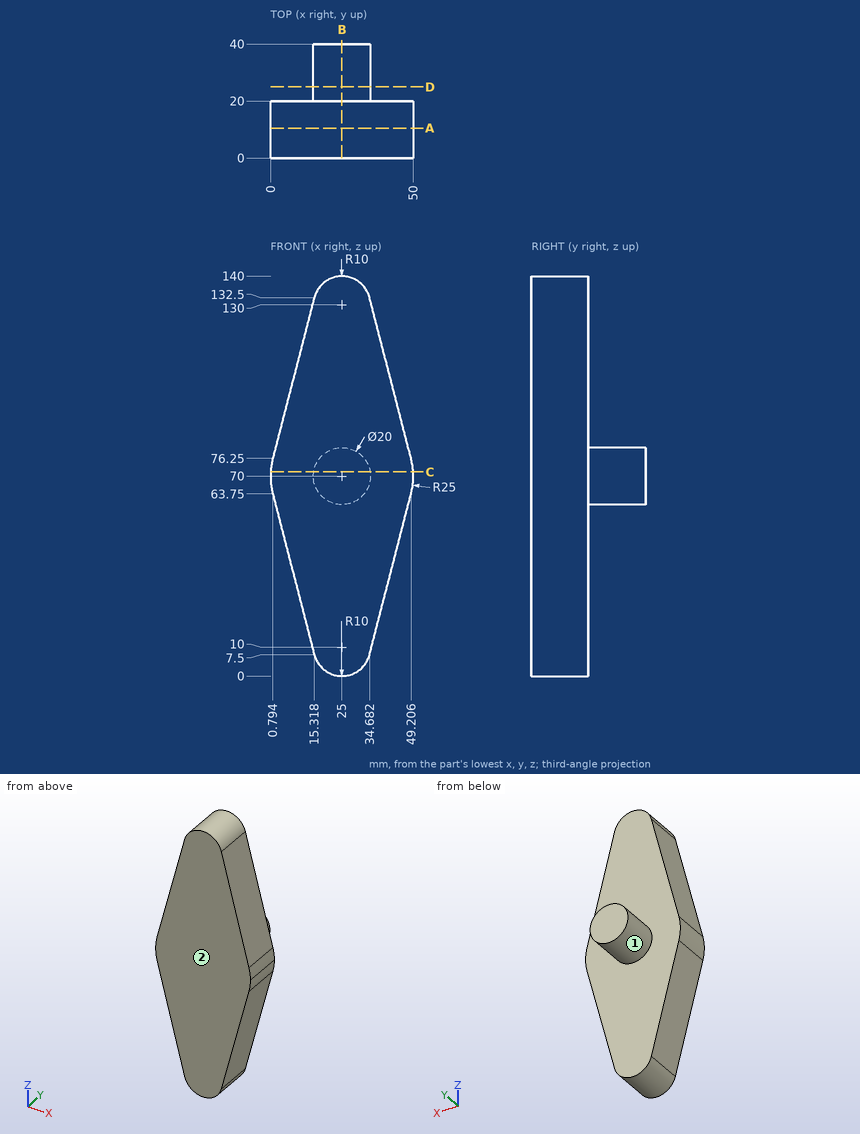
Here's the drawing with two shaded views (mm, measured from the low corner). I have some questions. A direction names the side the tool comes from. Round coordinates to 2 decimals unless told otherwise and drop trailing zeros. Loops run counter-clockwise (first coordinate to the right, second up) from the corner with the lowest first, then second, coordinate; pieces in that order, holes last.
Item 1: Suppose I cut it at A-A, the plane y = 10.5. Write out the boundary of the cut face in (x, z).
Item 2: Will these pins go through, and if not, where does the flat tip stop? pin 1 Ø1.5 at (x, z) = (15, 46.5) entering from -Y; pin 2 Ø6 at (y, z) = (16.5, 108) entering from +X; pin 3 Ø1.5 at (x, y) = (15.5, 30) entering from -Z; pin 4 Ø2 at (y, z) = (15, 23.5) entering from +X.
Item 3: Suppose I cut it at B-B, the plane x = 25. Write out the boundary of the cut face in (y, z), then the cut area to 3 significant figures.
Item 4: Suppose I cut it at C-C, the plane z = 71.5. Write out the boundary of the cut face in (x, y) (1 decimal), then the cut area to 3 significant figures.
Item 5: Which directions (+Z, -Z, +X, -X, +Y, -Y) give clear straight access to the entire face, cutting with the end or side of a thin tool? Please do the marked faces 1 and 2.
Item 6: Please list where these lines run through material, in increasing order: L1, parallel to Y at x = 11.5, z = 94.5; L2, parallel to Z at x = 20, y = 33; L3, parallel to X at y = 3, z = 65 (1 decimal).
Item 7: Suppose I cut it at D-D, the plane y = 25. Write out the boundary of the cut face in (x, z).
Reported:
1. outline: (0.79, 63.75) - (15.32, 7.5) arc R10 ccw to (34.68, 7.5) - (49.21, 63.75) arc R25 ccw to (50, 70) arc R25 ccw to (49.21, 76.25) - (34.68, 132.5) arc R10 ccw to (15.32, 132.5) - (0.79, 76.25) arc R25 ccw to start
2. pin 1: stops at y = 0
2. pin 2: stops at x = 41.78
2. pin 3: stops at z = 65.16
2. pin 4: stops at x = 39.07
3. outline: (0, 0) - (20, 0) - (20, 60) - (40, 60) - (40, 80) - (20, 80) - (20, 140) - (0, 140) - close
3. area: 3,200 mm2
4. outline: (0, 0) - (50, 0) - (50, 20) - (34.9, 20) - (34.9, 40) - (15.1, 40) - (15.1, 20) - (0, 20) - close
4. area: 1,390 mm2
5. face 1: +Y
5. face 2: +Z, -Z, +X, -X, -Y
6. L1: y = 0 to 20
6. L2: z = 61.34 to 78.66
6. L3: x = 0.5 to 49.5
7. outline: circle Ø20 at (25, 70)
